```python
from build123d import *

# Parameters (mm, degrees)
F0_W      = 152.4
F0_H      = 114.3
F1_DEPTH  = 91.948
F2_W      = 91.948
F2_H      = 101.6
F3_DEPTH  = 37.084
F4_W      = 91.948
F4_H      = 101.6
F5_DEPTH  = 37.084
F6_DEPTH  = 24.13
F7_DEPTH  = 25.4
F8_DEPTH  = 25.4
F9_DEPTH  = 25.4
F12_DEPTH = 86.36


with BuildPart() as f1:
    # F0 (on Front) → F1 (new body)
    with BuildSketch(Plane.XZ):
        Rectangle(F0_W, F0_H)
    extrude(amount=-F1_DEPTH)

    # F2 (on face) → F3 (cut)
    with BuildSketch(Plane.YZ.offset(76.2)):
        with Locations((45.974, 6.35)):
            Rectangle(F2_W, F2_H)
    extrude(amount=-F3_DEPTH, mode=Mode.SUBTRACT)

    # F4 (on face) → F5 (cut)
    with BuildSketch(Plane(origin=(-76.2, 0, 0), x_dir=(0, -1, 0), z_dir=(-1, 0, 0))):
        with Locations((-45.974, 6.35)):
            Rectangle(F4_W, F4_H)
    extrude(amount=-F5_DEPTH, mode=Mode.SUBTRACT)

    # F6 (add): a face of the model
    f6_faces = [f1.faces().sort_by_distance(p)[0] for p in [
        (39.116, 45.974, 6.35),
    ]]
    extrude(f6_faces, amount=F6_DEPTH)

    # F7 (add): a face of the model
    f7_faces = [f1.faces().sort_by_distance(p)[0] for p in [
        (-39.116, 45.974, 6.35),
    ]]
    extrude(f7_faces, amount=F7_DEPTH)

    # F8 (add): a face of the model
    f8_faces = [f1.faces().sort_by_distance(p)[0] for p in [
        (76.2, 45.974, -50.8),
    ]]
    extrude(f8_faces, amount=F8_DEPTH)

    # F9 (add): a face of the model
    f9_faces = [f1.faces().sort_by_distance(p)[0] for p in [
        (-76.2, 45.974, -50.8),
    ]]
    extrude(f9_faces, amount=F9_DEPTH)

    # F11 (on face) → F12 (cut)
    with BuildSketch(Plane(origin=(0, 0, -57.15), x_dir=(1, 0, 0), z_dir=(0, 0, -1))):
        Polygon((50.8, -69.2191192026), (50.8, -23.2451192026), (-50.8, -23.2451192026), (-50.8, -69.2191192026), (0, -69.2191192026), align=None)
    extrude(amount=-F12_DEPTH, mode=Mode.SUBTRACT)


solid = f1.part
```
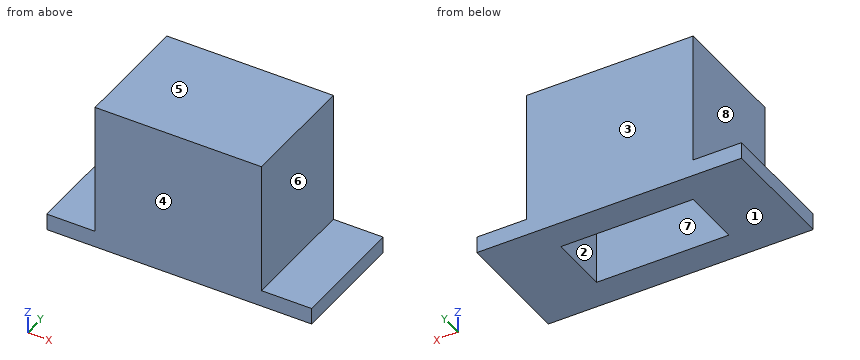
CAD build for the part. Positions are in the model's coordinates, mm. Face numbers are marked on the shaded views. A direction names the side the tool comes from. Round coordinates to 2 decimals unless told otherwise and drop trailing zeros. Loops run counter-clockwise (first coordinate to the right, second up) from the corner with the lowest first, then second, coordinate; pieces in that order, holes last. Notation, with made-up numbers: M -7,26 L 2,26 A25 ccw 2,53 Z; hole C 76.5,-31 d8. An arc over 180 degrees is marked long. Return JSON: item names as keys, results as strings. Group by question number.
(1) Wall check: probe 1 along Y at (x, z) = (-38, -2); probe 2 along X at (y, z) = (65, -44); probe 3 along Z at (x, y) = (93.5, 62). Give the ranges that are in metal, low to high. Write a range as [from, to].
(2) Saw through at A-A, the plane z = -49. List the corners of the cut face in (x, y).
(3) Saw through at D-D, the plane y = 29.5. List the corners of the cut face in (x, z).
(4) Mould opens along Y. For the marked faces 1, 2 and 3 say: +Y half, -Y half, draft (parallel to the pull), parting line (faces both ways), or undercut.
(5) Tool access for the marked faces 4, 5, 6, 7 and 8: list every direction of +Z, -Z, +X, -X, +Y, -Y with a clear straight run to the whole face (end or side of a thin tool).
(6) Saw through at B-B, the plane x = -41. List the corners of the cut face in (y, z), and give its area (3 significant figures).
(7) Drop flat-ended pins along their axis: P1, Ø1, axis at y = 71.5, z = -41, coming from the +X side; P2, Ø8, axis at y = 70.5, z = -30.5, coming from the -X side; P3, Ø19, axis at x = 83, y = 64.5, coming from the +Z side. Give the stop position or say it passes through.
(8) Saw through at C-C, the plane y = 81. List the corners of the cut face in (x, z).
Answer list:
{
 "1": {"probe 1": "[0, 23.25], [69.22, 91.95]", "probe 2": "[-64.52, -50.8], [50.8, 63.25]", "probe 3": "[-57.15, -44.45]"},
 "2": {"outline": "M -101.6,0 L 101.6,0 L 101.6,91.95 L -101.6,91.95 Z; hole M -50.8,23.25 L 50.8,23.25 L 50.8,69.22 L -50.8,69.22 Z"},
 "3": {"outline": "M -101.6,-57.15 L -50.8,-57.15 L -50.8,29.21 L 50.8,29.21 L 50.8,-57.15 L 101.6,-57.15 L 101.6,-44.45 L 63.25,-44.45 L 63.25,57.15 L -64.52,57.15 L -64.52,-44.45 L -101.6,-44.45 Z"},
 "4": {"face 1": "draft", "face 2": "undercut", "face 3": "+Y half"},
 "5": {"face 4": "+Z, -Z, +X, -X, -Y", "face 5": "+Z, +X, -X, +Y, -Y", "face 6": "+Z, +X, +Y, -Y", "face 7": "-Z", "face 8": "+Z, -X, +Y, -Y"},
 "6": {"outline": "M 0,-57.15 L 23.25,-57.15 L 23.25,29.21 L 69.22,29.21 L 69.22,-57.15 L 91.95,-57.15 L 91.95,57.15 L 0,57.15 Z", "area": "6,540 mm2"},
 "7": {"P1": "x = 63.25", "P2": "x = -64.52", "P3": "z = -44.45"},
 "8": {"outline": "M -101.6,-57.15 L 101.6,-57.15 L 101.6,-44.45 L 63.25,-44.45 L 63.25,57.15 L -64.52,57.15 L -64.52,-44.45 L -101.6,-44.45 Z"}
}
